Input: part model. Units: mm. Frame: model coordinates. Give positions to 0.01 mm unless a question says otherwise; leave off trailing zeros. Loops run counter-clockwise (first coordinate to the right, second up) from the corner with the lowest first, then second, coordinate; pieces in that order, holes last. Notation, with made-up numbers: M -9.5,-15 L 10.5,-15 A32 cw 10.5,24 Z; hole C -18.75,62 d6. An arc over 180 degrees is marked long. One line per item, written item: value. Start each with the question number.
(1) Ray query, line 1 along Y through (x, z) = (90, 5.5); line 2 along Y through (x, z) = (90, 0.8). Return the intervals inside material, ascending. Write a range as from..to.
(2) Section A-A on y = 0. Output: boundary loops of the cut face in (x, z).
(3) Pin query (flat end, axial travel): P1, Ø8, axis at x = -90, y = -90, coming from the -Z side; P2, Ø14.5, axis at x = 90, y = -90, coming from the -Z side. Return the tip coordinate at first contact, or that it passes through.
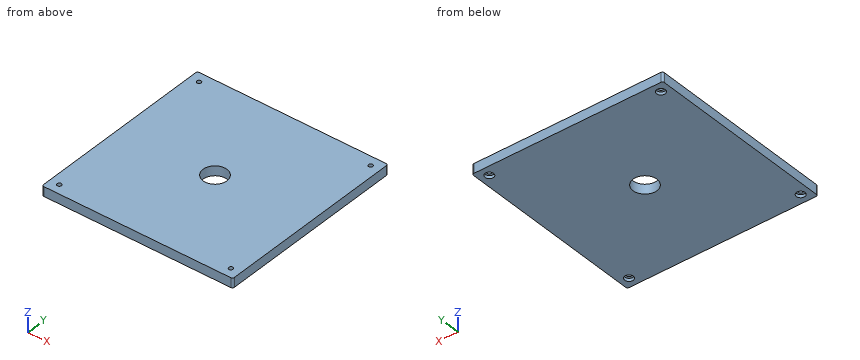
```python
from build123d import *

# Parameters (mm, degrees)
ESQUISSE1_R                                = 12.5
BOSS_EXTRU_1_DEPTH                         = 10
D_GAGEMENT_M41_D                           = 4.5
CHAMBRAGE_POUR_VIS_T_TE_RONDE_BOMB_2_COUNT = 2
CHAMBRAGE_POUR_VIS_T_TE_RONDE_BOMB_2_PITCH = 180
CHAMBRAGE_POUR_VIS_T_TE_RONDE_BOMB_3_COUNT = 2
CHAMBRAGE_POUR_VIS_T_TE_RONDE_BOMB_3_PITCH = 254.558441227
CHAMBRAGE_POUR_VIS_T_TE_RONDE_BOMB_4_COUNT = 2
CHAMBRAGE_POUR_VIS_T_TE_RONDE_BOMB_4_PITCH = 180


with BuildPart() as part:
    # Esquisse1 → Boss.-Extru.1 (new body)
    with BuildSketch(Plane.XY):
        with BuildLine():
            Line((-98, -100), (98, -100))
            ThreePointArc((98, -100), (99.414213562, -99.414213562), (100, -98))
            Line((100, -98), (100, 98))
            ThreePointArc((100, 98), (99.414213562, 99.414213562), (98, 100))
            Line((98, 100), (-98, 100))
            ThreePointArc((-98, 100), (-99.414213562, 99.414213562), (-100, 98))
            Line((-100, 98), (-100, -98))
            ThreePointArc((-100, -98), (-99.414213562, -99.414213562), (-98, -100))
        make_face()
        Circle(ESQUISSE1_R, mode=Mode.SUBTRACT)
    extrude(amount=BOSS_EXTRU_1_DEPTH)

    # Dégagement M41 (through all)
    with Locations(Plane.XY.offset(10)):
        with Locations((-90, 90), (-90, -90), (90, -90), (90, 90)):
            Hole(D_GAGEMENT_M41_D / 2)

    # Esquisse6 → Chambrage pour vis à tête ronde bombée M41 (revolve, cut)
    with BuildSketch(Plane(origin=(90, 90, 0), x_dir=(0, 1, 0), z_dir=(1, 0, 0))):
        Polygon((0, 0), (0, 10), (2.25, 10), (2.25, 3.125), (2.275, 3.1), (4.5, 3.1), (4.5, 0), align=None)
    chambrage_pour_vis_t_te_ronde_bomb_e_m = revolve(axis=Axis((90, 90, -6.35), (0, 0, 1)), mode=Mode.SUBTRACT)

    # Chambrage pour vis _ t_te ronde bomb 2: Chambrage pour vis à tête ronde bombée M41 ×2
    with Locations(*[(-i * CHAMBRAGE_POUR_VIS_T_TE_RONDE_BOMB_2_PITCH, 0, 0) for i in range(1, CHAMBRAGE_POUR_VIS_T_TE_RONDE_BOMB_2_COUNT)]):
        add(chambrage_pour_vis_t_te_ronde_bomb_e_m, mode=Mode.SUBTRACT)

    # Chambrage pour vis _ t_te ronde bomb 3: Chambrage pour vis à tête ronde bombée M41 ×2
    with Locations(*[Vector(-0.7071067811865476, -0.7071067811865476, 0) * (i * CHAMBRAGE_POUR_VIS_T_TE_RONDE_BOMB_3_PITCH) for i in range(1, CHAMBRAGE_POUR_VIS_T_TE_RONDE_BOMB_3_COUNT)]):
        add(chambrage_pour_vis_t_te_ronde_bomb_e_m, mode=Mode.SUBTRACT)

    # Chambrage pour vis _ t_te ronde bomb 4: Chambrage pour vis à tête ronde bombée M41 ×2
    with Locations(*[(0, -i * CHAMBRAGE_POUR_VIS_T_TE_RONDE_BOMB_4_PITCH, 0) for i in range(1, CHAMBRAGE_POUR_VIS_T_TE_RONDE_BOMB_4_COUNT)]):
        add(chambrage_pour_vis_t_te_ronde_bomb_e_m, mode=Mode.SUBTRACT)


solid = part.part
```
Output values:
1. line 1: y = -100..-92.25, -87.75..87.75, 92.25..100
1. line 2: y = -100..-94.5, -85.5..85.5, 94.5..100
2. outline: M -100,0 L -12.5,0 L -12.5,10 L -100,10 Z; M 12.5,0 L 100,0 L 100,10 L 12.5,10 Z
3. P1: stops at z = 3.1
3. P2: stops at z = 0
